Design review of the part built by this model. Coordinates are the model's own, in mm. A direction names the side the tool comes from. Round coordinates to 2 decimals unless told otherwise and drop trailing zeros. Write each loop counter-clockwise with the first axis right and the second up, starting at its lowest first coordinate (ties: lowest second). Pieces come first, ordered by that corner, then holes. Notation, with made-up numbers: M 34.5,32 L 53.5,32 A15 ccw 53.5,60 Z; hole C 28.5,73 d3. An arc over 180 degrees is marked long. One line per question, with ' | ' between items. Start each with the question number.
Item 1: Add section D-D, the plane x = 9. State the section outline as (y, z) points (3 decimals), and give its area (3 significant figures).
Item 2: Draft analysis for pull direction X (two halves, no side actions). For faces 1 (the face through (4, -10.045, 0)), 2 (the face through (7, 0, -20)), 3 (the face through (-9.91, 0, 0)), state which applies: released by +X, released by -X, zero draft, split by the parting line, or undercut.
Item 3: Insertion check: pin 1 Ø13.5 at (x, z) = (9, 3) entering from +Y (3 decimals); pin 2 Ø13.5 at (x, z) = (69, -7.5) entering from -Y (3 decimals); pin 3 Ø6 at (x, y) = (13.5, 4) entering from -Z. Each pin has a flat end and moves straight along its axis. Give the tip position at first contact, or say it passes through.
Item 4: Add section A-A, the plane z = 9. State the section outline as (x, y) points (3 decimals), and give its area (3 significant figures).
Item 5: Add section C-C, the plane y = 0. State the section outline as (x, z) points, and give its area (3 significant figures).
Item 6: Add section B-B, the plane x = 78. State the section outline as (y, z) points (3 decimals), and give its area (3 significant figures).
Item 7: Machinability: for faces 4 (the face through (-5.158, -3.955, -22.514)), 5 (the face through (74, 10.045, 0)), 6 (the face through (4, 10.045, 0)), which of the approach directions +Z, -Z, +X, -X, +Y, -Y give a long, thin tool a straight path to every point of the face, cutting with its end or side? Answer none if there is none.
Item 8: For L1, parallel to Z at x = 46, y = -5.75; L2, parallel to Y at x = 15, z = -5 (3 decimals); L3, parallel to Z at x = 67, y = -3.75, list the stretches that pass through material, from the lowest coordinate up.
```python
from build123d import *

# Parameters (mm, degrees)
EXTRUDE_1_DEPTH      = 20
SKETCH_2_W           = 43
SKETCH_2_H           = 22
EXTRUDE_2_DEPTH      = 21
SKETCH_3_R           = 6.5
EXTRUDE_4_DEPTH      = 24.8
EXTRUDE_4_DEPTH_BACK = 25.1


with BuildPart() as part:
    # Эскиз1 → Бобышка-Вытянуть1 (new body, symmetric)
    with BuildSketch(Plane.XY):
        Polygon((17.5, -10.045), (17.5, -11.495), (60.5, -11.495), (60.5, -10.045), (87.91, -10.045), (87.91, 10.045), (60.5, 10.045), (60.5, 10.505), (17.5, 10.505), (17.5, 10.045), (-9.91, 10.045), (-9.91, -10.045), align=None)
    extrude(amount=EXTRUDE_1_DEPTH, both=True)

    # Эскиз2 → Бобышка-Вытянуть2 (add, symmetric)
    with BuildSketch(Plane.XY):
        with Locations((39, -0.495)):
            Rectangle(SKETCH_2_W, SKETCH_2_H)
    extrude(amount=EXTRUDE_2_DEPTH, both=True)

    # Эскиз3 → Бобышка-Вытянуть4 (add, two sides)
    with BuildSketch(Plane.XY) as extrude_4_sk:
        Circle(SKETCH_3_R)
        with Locations((78, 0)):
            Circle(SKETCH_3_R)
    extrude(amount=EXTRUDE_4_DEPTH)
    extrude(extrude_4_sk.sketch, amount=-EXTRUDE_4_DEPTH_BACK)


solid = part.part
```
Computed values:
1) outline: M -10.045,-20 L 10.045,-20 L 10.045,20 L -10.045,20 Z | area: 804 mm^2
2) face 1: zero draft | face 2: undercut | face 3: released by -X
3) pin 1: stops at y = 10.045 | pin 2: stops at y = -10.045 | pin 3: stops at z = -20
4) outline: M -9.91,-10.045 L 17.5,-10.045 L 17.5,-11.495 L 60.5,-11.495 L 60.5,-10.045 L 87.91,-10.045 L 87.91,10.045 L 60.5,10.045 L 60.5,10.505 L 17.5,10.505 L 17.5,10.045 L -9.91,10.045 Z | area: 2,050 mm^2
5) outline: M -9.91,-20 L -6.5,-20 L -6.5,-25.1 L 6.5,-25.1 L 6.5,-20 L 17.5,-20 L 17.5,-21 L 60.5,-21 L 60.5,-20 L 71.5,-20 L 71.5,-25.1 L 84.5,-25.1 L 84.5,-20 L 87.91,-20 L 87.91,20 L 84.5,20 L 84.5,24.8 L 71.5,24.8 L 71.5,20 L 60.5,20 L 60.5,21 L 17.5,21 L 17.5,20 L 6.5,20 L 6.5,24.8 L -6.5,24.8 L -6.5,20 L -9.91,20 Z | area: 4,260 mm^2
6) outline: M -10.045,-20 L -6.5,-20 L -6.5,-25.1 L 6.5,-25.1 L 6.5,-20 L 10.045,-20 L 10.045,20 L 6.5,20 L 6.5,24.8 L -6.5,24.8 L -6.5,20 L -10.045,20 Z | area: 932 mm^2
7) face 4: -Z | face 5: +Z, -Z, +X, +Y | face 6: +Z, -Z, -X, +Y
8) L1: z = -21 to 21 | L2: y = -10.045 to 10.045 | L3: z = -20 to 20
